from build123d import *

# Parameters (mm, degrees)
F1_DEPTH = 25.4
F2_DEPTH = 25.4


with BuildPart() as f1:
    # F0 (on Front) → F1 (new body)
    with BuildSketch(Plane.XZ):
        with BuildLine():
            ThreePointArc((-29.4565436219, 23.8478247362), (-34.2387511178, 12.3025545416), (-45.7840213124, 7.5203470458))
            Line((-45.7840213124, 7.5203470458), (-45.7840213124, -23.8478247362))
            Line((-45.7840213124, -23.8478247362), (-3.5301e-06, -23.8478247362))
            ThreePointArc((-3.5301e-06, -23.8478247362), (2.0304351181, -21.7171458616), (3.8633102693, -19.4143123352))
            ThreePointArc((3.8633102693, -19.4143123352), (-19.7949662714, 0), (3.8633102693, 19.4143123352))
            ThreePointArc((3.8633102693, 19.4143123352), (2.0304351181, 21.7171458616), (-3.5301e-06, 23.8478247362))
            Line((-3.5301e-06, 23.8478247362), (-29.4565436219, 23.8478247362))
        make_face()
    extrude(amount=F1_DEPTH)

    # F0 (on Front) → F2 (join)
    with BuildSketch(Plane.XZ):
        with BuildLine():
            Line((45.7840142522, 23.8478247362), (-3.5301e-06, 23.8478247362))
            ThreePointArc((-3.5301e-06, 23.8478247362), (2.0304351181, 21.7171458616), (3.8633102693, 19.4143123352))
            ThreePointArc((3.8633102693, 19.4143123352), (15.3022022298, 12.5572009861), (19.7949662714, 0))
            ThreePointArc((19.7949662714, 0), (15.3022022298, -12.5572009861), (3.8633102693, -19.4143123352))
            ThreePointArc((3.8633102693, -19.4143123352), (2.0304351181, -21.7171458616), (-3.5301e-06, -23.8478247362))
            Line((-3.5301e-06, -23.8478247362), (45.7840283725, -23.8478247362))
            Line((45.7840283725, -23.8478247362), (45.7840241128, -9.4592027554))
            add(Edge.make_bspline(
                [(45.784018512, 9.4592027554), (21.3751961487, 9.4592016702), (21.3751989491, -1.0852e-06), (21.3752017495, -9.4592038407), (45.7840241128, -9.4592027554)],
                knots=[1.5707964415, 1.5707964415, 1.5707964415, 3.1415927683, 3.1415927683, 4.7123890951, 4.7123890951, 4.7123890951], degree=2, weights=[1, 0.7071067812, 1, 0.7071067812, 1]))
            Line((45.784018512, 9.4592027554), (45.7840142522, 23.8478247362))
        make_face()
    extrude(amount=F2_DEPTH)


solid = f1.part
Part model, mm, in its own coordinate system. Give positions to 0.01 mm unless a question says otherwise; leave off trailing zeros. Order: outer loops, then holes, each group sorted by start corner. A loop starts at its lowest first (then second) coordinate and runs counter-clockwise, first axis right, second up. Notation, with made-up numbers: (6, 1) - (14, 1) arc R25 ccw to (14, 16) - close; hole circle Ø3 at (-8, 35). An arc over 180 degrees is marked (long way). Use a Markdown table: item, result.
1) Probe L1, parallel to Z at x = 0, y = -19.5; L2, parallel to X at y = -8, z = 0; L3, parallel to Z at x = -8.5, y = -24.25. List the from-to ranges inside material, lowest first. Write a range as from..to.
Checked values:
| item | result |
|---|---|
| L1 | -23.85..-19.79, 19.79..23.85 |
| L2 | -45.78..-19.79, 19.79..21.38 |
| L3 | -23.85..-17.88, 17.88..23.85 |
2) Saw through at B-B on z = -11.5. List the corners of the cut face in (x, y), plus the area to 3 significant figures.
Checked values:
| item | result |
|---|---|
| outline | (-45.78, -25.4) - (-16.11, -25.4) - (-16.11, 0) - (-45.78, 0) - close; (16.11, -25.4) - (45.78, -25.4) - (45.78, 0) - (16.11, 0) - close |
| area | 1,510 mm² |
3) Saw through at A-A on x = 0. List the corners of the cut face in (y, z), plus the area to 3 significant figures.
Checked values:
| item | result |
|---|---|
| outline | (-25.4, -23.85) - (0, -23.85) - (0, -19.79) - (-25.4, -19.79) - close; (-25.4, 19.79) - (0, 19.79) - (0, 23.85) - (-25.4, 23.85) - close |
| area | 206 mm² |
